For this review, take the finished solid that the model builds, in its own axes (mm). A direction names the side the tool comes from. Give positions to 0.01 mm unless a question says otherwise; leave off trailing zeros. Order: outer loops, then holes, each group sorted by start corner. A loop starts at its lowest first (then second) coordinate and runs counter-clockwise, first axis right, second up. Notation, with made-up numbers: (74, 37.25) - (82, 37.25) arc R18 ccw to (82, 43.25) - close; hole circle Ø1 at (45, 24.5). An arc over 180 degrees is marked (long way). Put each result on its own line as item: value. Start each with the question number.
```python
from build123d import *

# Parameters (mm, degrees)
F0_R     = 12.7
F1_DEPTH = 101.6
F2_R     = 5.08


with BuildPart() as f1:
    # F0 (on Front) → F1 (new body)
    with BuildSketch(Plane.XZ):
        Polygon((29.100048, 119.942114), (-47.099952, 119.942114), (-47.099952, -57.857886), (29.100048, -57.857886), (29.100048, -32.457886), (3.700048, -32.457886), (3.700048, 94.542114), (29.100048, 94.542114), align=None)
        with Locations((-21.699952, -32.457886)):
            Circle(F0_R, mode=Mode.SUBTRACT)
        with Locations((-21.699952, 5.642114)):
            Circle(F0_R, mode=Mode.SUBTRACT)
        with Locations((-21.699952, 56.442114)):
            Circle(F0_R, mode=Mode.SUBTRACT)
        with Locations((-21.699952, 94.542114)):
            Circle(F0_R, mode=Mode.SUBTRACT)
    extrude(amount=F1_DEPTH)

    # F2
    f2_edges = [f1.edges().sort_by_distance(p)[0] for p in [
        (-8.999952, -101.6, 119.942114),
        (-47.099952, -101.6, 31.042114),
        (29.100048, -101.6, 107.242114),
        (16.400048, -101.6, 94.542114),
        (3.700048, -101.6, 31.042114),
        (16.400048, -101.6, -32.457886),
        (29.100048, -101.6, -45.157886),
        (-8.999952, -101.6, -57.857886),
        (-47.099952, -50.8, 119.942114),
        (-8.999952, 0, 119.942114),
        (29.100048, -50.8, 119.942114),
        (-47.099952, 0, 31.042114),
        (-47.099952, -50.8, -57.857886),
        (29.100048, -50.8, -32.457886),
        (3.700048, -50.8, -32.457886),
        (29.100048, -50.8, 94.542114),
        (29.100048, 0, 107.242114),
        (29.100048, -50.8, -57.857886),
        (29.100048, 0, -45.157886),
        (3.700048, -50.8, 94.542114),
        (16.400048, 0, 94.542114),
        (3.700048, 0, 31.042114),
        (16.400048, 0, -32.457886),
        (-8.999952, 0, -57.857886),
    ]]
    fillet(f2_edges, radius=F2_R)


solid = f1.part
```
1. Add section C-C, the plane z = -4. Give the boundary of the cut face in (x, y).
2. Wall thickness on line 1 (Z direction, x = 8.5, y = -71); line 2 (Z direction, x = 11, y = -47); line 3 (Z direction, x = -31, y = -32): over which ranges is each line inside the solid? List them lowest first. Write a range as from..to.
3. Add section D-D, the plane y = -67.5. Give the boundary of the cut face in (x, z), then the cut area to 3 significant figures.
4. Tool access review of faces 4 (the face through (-45.65, -51.44, -56.33)), 5 (the face through (2.251, -1.528, 31.86)), 6 (the face through (27.65, -51.44, 96.07)): name each direction out of +Z, -Z, +X, -X, +Y, -Y from which nothing blocks a thin tool from reaching the whole face with its end or side.
5. Add section A-A, the plane x = -20.5. Give the boundary of the cut face in (y, z), then the cut area to 3 significant figures.
6. Clearance check with flat-ended pins moving along their axes: pin 1 (12 mm diameter, centred on y = -11.5, z = 7, fed in from +X); pin 2 (20.5 mm diameter, centred on x = -21.7, z = 94.54, fed in from +Y). State where each tip first meets the part, or that it passes through.
7. Add section B-B, the plane z = 72.5. Give the boundary of the cut face in (x, y), then the cut area to 3 significant figures.
8. The part is to be moulded in two halves that separate along Z. For faces 1 (the face through (16, -50, 94.542)), 2 (the face through (29.1, -50, 107)), 3 (the face through (-9, -50, 119.942)), say which applies: released by +Z, released by -Z, zero draft, split by the parting line, or undercut.
Found:
1. outline: (-47.1, -96.52) arc R5.08 ccw to (-42.02, -101.6) - (-29.97, -101.6) - (-29.97, 0) - (-42.02, 0) arc R5.08 ccw to (-47.1, -5.08) - close; (-13.43, -101.6) - (-1.38, -101.6) arc R5.08 ccw to (3.7, -96.52) - (3.7, -5.08) arc R5.08 ccw to (-1.38, 0) - (-13.43, 0) - close
2. line 1: z = -57.86..-32.45, 94.53..119.94
2. line 2: z = -57.86..-32.46, 94.54..119.94
2. line 3: z = -57.86..-41.11, -23.81..-3.01, 14.29..47.79, 65.09..85.89, 103.19..119.94
3. outline: (-47.1, -52.78) arc R5.08 ccw to (-42.02, -57.86) - (24.02, -57.86) arc R5.08 ccw to (29.1, -52.78) - (29.1, -37.54) arc R5.08 ccw to (24.02, -32.46) - (8.78, -32.46) arc R5.08 cw to (3.7, -27.38) - (3.7, 89.46) arc R5.08 cw to (8.78, 94.54) - (24.02, 94.54) arc R5.08 ccw to (29.1, 99.62) - (29.1, 114.86) arc R5.08 ccw to (24.02, 119.94) - (-42.02, 119.94) arc R5.08 ccw to (-47.1, 114.86) - close; hole circle Ø25.4 at (-21.7, -32.46); hole circle Ø25.4 at (-21.7, 5.64); hole circle Ø25.4 at (-21.7, 56.44); hole circle Ø25.4 at (-21.7, 94.54)
3. area: 8,270 mm^2
4. face 4: -Z, -X, +Y, -Y
4. face 5: +X, +Y
4. face 6: +X, +Y, -Y
5. outline: (-101.6, -52.78) arc R5.08 ccw to (-96.52, -57.86) - (-5.08, -57.86) arc R5.08 ccw to (0, -52.78) - (0, -45.1) - (-101.6, -45.1) - close; (-101.6, -19.81) - (0, -19.81) - (0, -7) - (-101.6, -7) - close; (-101.6, 18.29) - (0, 18.29) - (0, 43.8) - (-101.6, 43.8) - close; (-101.6, 69.09) - (0, 69.09) - (0, 81.9) - (-101.6, 81.9) - close; (-101.6, 107.19) - (0, 107.19) - (0, 114.86) arc R5.08 ccw to (-5.08, 119.94) - (-96.52, 119.94) arc R5.08 ccw to (-101.6, 114.86) - close
5. area: 7,770 mm^2
6. pin 1: stops at x = 3.7
6. pin 2: passes through
7. outline: (-47.1, -96.52) arc R5.08 ccw to (-42.02, -101.6) - (-1.38, -101.6) arc R5.08 ccw to (3.7, -96.52) - (3.7, -5.08) arc R5.08 ccw to (-1.38, 0) - (-42.02, 0) arc R5.08 ccw to (-47.1, -5.08) - close
7. area: 5,140 mm^2
8. face 1: undercut
8. face 2: zero draft
8. face 3: released by +Z
